Source: CAD feature listing. Evaluate the final solid. Frame: model axes, mm. A direction names the side the tool comes from. Round coordinates to 2 decimals unless told otherwise and drop trailing zeros. Order: outer loops, then holes, each group sorted by start corner. A loop starts at its lowest first (then second) coordinate and runs counter-clockwise, first axis right, second up. Notation, with made-up numbers: (36, 26) -> (75, 26) arc R32 ccw to (75, 53) -> close; hole circle Ø4 at (86, 28). An arc over 180 degrees is marked (long way). Answer as CSV lines item,"result".
from build123d import *

# Parameters (mm, degrees)
SKETCH_W     = 8
SKETCH_H     = 6.5
PAD_DEPTH    = 2
SKETCH001_W  = 5.1
SKETCH001_H  = 1.9
PAD001_DEPTH = 1.4


with BuildPart() as part:
    # Sketch → Pad (new body)
    with BuildSketch(Plane.XZ):
        with Locations((4, 3.25)):
            Rectangle(SKETCH_W, SKETCH_H)
    extrude(amount=PAD_DEPTH)

    # Sketch001 (on Face6 of Pad) → Pad001 (join)
    with BuildSketch(Plane.XZ.offset(2)):
        with Locations((4.05, 1.95)):
            Rectangle(SKETCH001_W, SKETCH001_H)
    extrude(amount=PAD001_DEPTH)


solid = part.part
1. Pin query (flat end, axial travel): pin 1 (0.7 mm diameter, centred on x = 3.5, y = -3, fed in from +Z). Return the tip coordinate at first contact, or that it passes through.
Results below:
pin 1,"z = 2.9"
2. Line query: L1, parallel to Y at x = 4.75, z = 3; L2, parallel to Z at x = 4, y = -2.4; L3, parallel to X at y = -2.6, z = 2. Output: solid intervals per line, ascending. Write a range as [from, to].
Results below:
L1,"[-2, 0]"
L2,"[1, 2.9]"
L3,"[1.5, 6.6]"
3. Reachability of faces 1 (the flat face through (6.6, -3, 2)), 2 (the flat face through (4, 0, 3)), 3 (the flat face through (1.5, -3, 2)), 4 (the flat face through (4, -3, 1)), 5 (the flat face through (4, -3, 2.9)) from +Z, -Z, +X, -X, +Y, -Y: full face, straight path, thin tool, end or side. Return the list, or none.
Results below:
face 1,"+Z, -Z, +X, -Y"
face 2,"+Z, -Z, +X, -X, +Y"
face 3,"+Z, -Z, -X, -Y"
face 4,"-Z, +X, -X, -Y"
face 5,"+Z, +X, -X, -Y"
4. Section query A-A on z = 2.5. Return loops of the section in (x, y), and give its area (3 significant figures).
Results below:
outline,"(0, -2) -> (1.5, -2) -> (1.5, -3.4) -> (6.6, -3.4) -> (6.6, -2) -> (8, -2) -> (8, 0) -> (0, 0) -> close"
area,"23.1 mm2"
5. Section query C-C on y = -2.9. Return loops of the section in (x, z).
Results below:
outline,"(1.5, 1) -> (6.6, 1) -> (6.6, 2.9) -> (1.5, 2.9) -> close"
6. Section query B-B on x = 4.5. Return loops of the section in (y, z), and give its area (3 significant figures).
Results below:
outline,"(-3.4, 1) -> (-2, 1) -> (-2, 0) -> (0, 0) -> (0, 6.5) -> (-2, 6.5) -> (-2, 2.9) -> (-3.4, 2.9) -> close"
area,"15.7 mm2"
7. Section query D-D on x = 7. Return loops of the section in (y, z).
Results below:
outline,"(-2, 0) -> (0, 0) -> (0, 6.5) -> (-2, 6.5) -> close"
